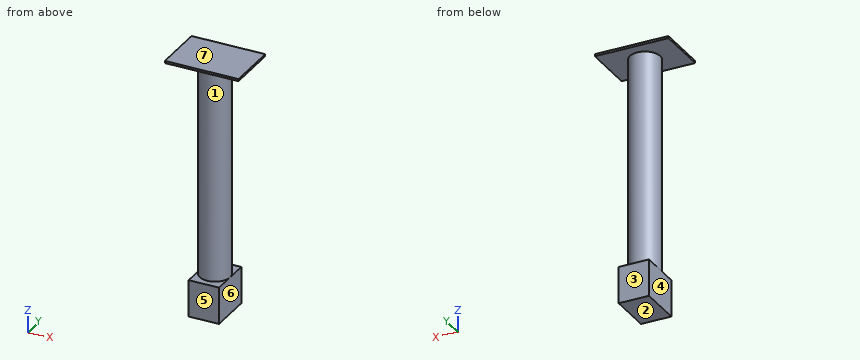
Autodesk Inventor part; units mm, degrees
ref_plane "YZ Plane" through (0, 0, 0) normal (1, 0, 0) x (0, 1, 0)
ref_plane "XZ Plane" through (0, 0, 0) normal (0, 1, 0) x (-1, 0, 0)
ref_plane "XY Plane" through (0, 0, 0) normal (0, 0, 1) x (1, 0, 0)
sketch "Sketch1" plane through (0, 0, 0) normal (0, 0, 1) x (1, 0, 0)
  circle A0 centre (0, 0) radius 7
  dimension "d0" = 14
extrude "Extrusion1" add sketch "Sketch1" along normal blind 100
sketch "Sketch2" plane through (0, 0, 0) normal (0, 0, -1) x (-1, 0, 0)
  circle A0 centre (0, 0) radius 6.4031
extrude "Extrusion2" cut sketch "Sketch2" against normal blind 1000
sketch "Sketch3" plane through (0, 0, 100) normal (0, 0, 1) x (1, 0, 0)
  line L0 (17, -12) -> (-17, -12)
  line L1 (-17, -12) -> (-17, 12)
  line L2 (-17, 12) -> (17, 12)
  line L3 (17, 12) -> (17, -12)
  point P0 (0, 0)
  dimension "d5" = 34
  dimension "d6" = 24
extrude "Extrusion3" add sketch "Sketch3" along normal blind 1
sketch "Sketch4" plane through (0, 0, 0) normal (0, 0, -1) x (-1, 0, 0)
  line L0 (7, -10) -> (-7, -10)
  line L1 (-7, -10) -> (-7, 10)
  line L2 (-7, 10) -> (7, 10)
  line L3 (7, 10) -> (7, -10)
  point P0 (0, 0)
  dimension "d9" = 14
  dimension "d10" = 20
extrude "Extrusion4" add sketch "Sketch4" along normal blind 17
properties part number "muñeca eje"
Verification items for the finished model (mm, model axes). Face numbers are marked on the shaded views. A direction names the side the tool comes from. Give positions to 0.01 mm unless a question says otherwise; leave off trailing zeros. Write each loop counter-clockwise with the first axis right and the second up, starting at its lowest first coordinate (ties: lowest second). Pieces come first, ordered by that corner, then holes. Notation, with made-up numbers: M 48.25,-33.75 L 57.25,-33.75 A28 cw 57.25,-3.75 Z; hole C -24,-20 d5. An arc over 180 degrees is marked long. Write item = value, one per line.
(1) Sectioned sample at B-B (y = -3). Record the cut outline in (x, z), then the cut area to 3 significant figures.
Found:
outline = M -17,100 L -6.32,100 L -6.32,0 L -7,0 L -7,-17 L 7,-17 L 7,0 L 6.32,0 L 6.32,100 L 17,100 L 17,101 L -17,101 Z; hole M -5.66,0 L 5.66,0 L 5.66,100 L -5.66,100 Z
area = 406 mm2
(2) Sectioned sample at D-D (x = -10). Record the cut outline in (y, z), then the cut area to 3 significant figures.
Found:
outline = M -12,100 L 12,100 L 12,101 L -12,101 Z
area = 24.0 mm2
(3) Access from +Z, -Z, +X, -X, +Y, -Y to the whole of each face (thin tool, end or side, straight path). Record for the marked faces 4, 5, 6 and 7.
Found:
face_4 = -Z, -X, +Y, -Y
face_5 = -Z, +X, -X, -Y
face_6 = -Z, +X, +Y, -Y
face_7 = +Z, +X, -X, +Y, -Y
(4) Go/stop test with flat-tipped pins: pin 1 Ø2 at (x, z) = (-8.5, 75) entering from +Y; pin 2 Ø6 at (x, z) = (-5.5, 65) entering from -Y; pin 3 Ø12 at (y, z) = (3, 88.5) entering from -X; pin 4 Ø8 at (x, z) = (1.5, 11) entering from +Y. Record where each tip stops, or that it passes through.
Found:
pin_1 = through
pin_2 = -6.54
pin_3 = -7
pin_4 = 7
(5) Material ranges on line 1 (Z direction, x = 4, y = -2.5); line 2 (Y direction, x = 0, z = 27); line 3 (Z direction, x = -2, y = 10.25), recorded low to high.
Found:
line_1 = -17 to 0, 100 to 101
line_2 = -7 to -6.4, 6.4 to 7
line_3 = 100 to 101
(6) Sectioned sample at C-C (z = 46). Record the cut outline in (x, y).
Found:
outline = C 0,0 d14; hole C 0,0 d12.81
(7) Draft check along Z on the marked faces 1, 2 and 3. Enter one of: released by +Z, released by -Z, zero draft, split by the parting line, or undercut.
Found:
face_1 = undercut
face_2 = released by -Z
face_3 = zero draft
(8) Sectioned sample at A-A (x = 0). Record the cut outline in (y, z), then the cut area to 3 significant figures.
Found:
outline = M -12,100 L -7,100 L -7,0 L -10,0 L -10,-17 L 10,-17 L 10,0 L 7,0 L 7,100 L 12,100 L 12,101 L -12,101 Z; hole M -6.4,0 L 6.4,0 L 6.4,100 L -6.4,100 Z
area = 483 mm2
